Model file for the job. Use its own axes, mm. Face numbers are marked on the shaded views. Give positions to 0.01 mm unless a question says otherwise; leave off trailing zeros. Write each loop counter-clockwise with the first axis right and the second up, starting at its lowest first coordinate (ties: lowest second). Pieces come first, ordered by that corner, then holes. Notation, with made-up numbers: (-20, -15.75) - (15, -15.75) arc R27 ccw to (15, 10.25) - close; hole circle Ø9 at (0, 83). An arc over 180 degrees is marked (long way). Use CSV: the item, a comma, the result in double quotes.
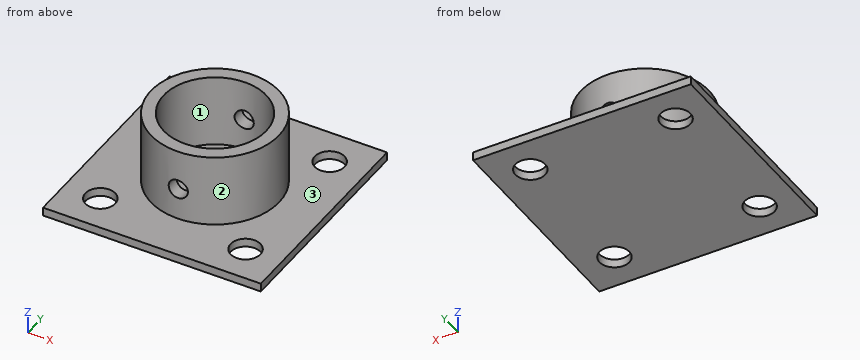
from build123d import *

# Parameters (mm, degrees)
F0_W     = 51
F0_H     = 51
F0_R     = 3.5
F1_DEPTH = 2
F2_R     = 15
F2_R_2   = 12
F3_DEPTH = 17
F4_W     = 51
F4_H     = 2.453923
F5_DEPTH = 17
F6_R     = 2.25
F7_DEPTH = 51.001
F8_W     = 51
F8_H     = 2.453923
F9_DEPTH = 17


with BuildPart() as f1:
    # F0 (on Top) → F1 (new body)
    with BuildSketch(Plane.XY):
        with Locations((-30.284861, 20.886204)):
            Rectangle(F0_W, F0_H)
        with Locations((-47.284861, 3.886204)):
            Circle(F0_R, mode=Mode.SUBTRACT)
        with Locations((-13.284861, 3.886204)):
            Circle(F0_R, mode=Mode.SUBTRACT)
        with Locations((-47.284861, 37.886204)):
            Circle(F0_R, mode=Mode.SUBTRACT)
        with Locations((-13.284861, 37.886204)):
            Circle(F0_R, mode=Mode.SUBTRACT)
    extrude(amount=F1_DEPTH)

    # F2 (on face) → F3 (join)
    with BuildSketch(Plane.XY.offset(2)):
        with Locations((-30.284861, 20.886204)):
            Circle(F2_R)
        with Locations((-30.284861, 20.886204)):
            Circle(F2_R_2, mode=Mode.SUBTRACT)
    extrude(amount=F3_DEPTH)

    # F4 (on face) → F5 (join)
    with BuildSketch(Plane.XY.offset(2)):
        with Locations((-30.284861, -3.386834)):
            Rectangle(F4_W, F4_H)
    extrude(amount=F5_DEPTH)

    # F6 (on face) → F7 (cut, through all)
    with BuildSketch(Plane.XZ.offset(4.613796)):
        with Locations((-30.284861, 9.5)):
            Circle(F6_R)
    extrude(amount=-F7_DEPTH, mode=Mode.SUBTRACT)

    # F8 (on face) → F9 (cut)
    with BuildSketch(Plane.XY.offset(19)):
        with Locations((-30.284861, -3.386834)):
            Rectangle(F8_W, F8_H)
    extrude(amount=-F9_DEPTH, mode=Mode.SUBTRACT)


solid = f1.part
(1) Saw through at B-B, the plane z = 9.5. List the corners of the cut face in (x, y), then the cut area to 3 significant figures.
Checked values:
outline,"(-32.53, 6.06) - (-32.53, 9.1) arc R12 cw to (-32.53, 32.67) - (-32.53, 35.72) arc R15 ccw to start; (-28.03, 6.06) arc R15 ccw to (-28.03, 35.72) - (-28.03, 32.67) arc R12 cw to (-28.03, 9.1) - close"
area,"227 mm^2"
(2) Saw through at C-C, the plane y = 1. List the corners of the cut face in (x, z) (3 decimals).
Checked values:
outline,"(-55.785, 0) - (-49.265, 0) - (-49.265, 2) - (-55.785, 2) - close; (-45.305, 0) - (-15.265, 0) - (-15.265, 2) - (-45.305, 2) - close; (-11.305, 0) - (-4.785, 0) - (-4.785, 2) - (-11.305, 2) - close"
(3) Saw through at A-A, the plane x = -29. List the corners of the cut face in (y, z).
Checked values:
outline,"(-4.61, 0) - (46.39, 0) - (46.39, 2) - (35.83, 2) - (35.83, 7.65) - (32.82, 7.65) - (32.82, 2) - (8.96, 2) - (8.96, 7.65) - (5.94, 7.65) - (5.94, 2) - (-4.61, 2) - close; (5.94, 11.35) - (8.96, 11.35) - (8.96, 19) - (5.94, 19) - close; (32.82, 11.35) - (35.83, 11.35) - (35.83, 19) - (32.82, 19) - close"
(4) Flat gauge pins, fed straight in: P1, Ø8, axis at x = -32, z = 8.5, coming from the +Y side; P2, Ø11, axis at x = -47.28, y = 37.89, coming from the +Z side. Where does each tip first touch, or does it go through?
Checked values:
P1,"stops at y = 35.89"
P2,"stops at z = 2"
(5) Wall check: probe 1 along X at (y, z) = (28, 7.5); probe 2 along Y at (x, z) = (-25, 8.5); probe 3 along Y at (x, z) = (-39, 6.25). Give the ranges that are in metal, low to high. Write a range as [from, to].
Checked values:
probe 1,"x = [-43.49, -39.95], [-20.62, -17.08]"
probe 2,"y = [6.85, 10.11], [31.66, 34.92]"
probe 3,"y = [8.68, 12.64], [29.14, 33.09]"
(6) Saw through at D-D, the plane y = 30.5. List the corners of the cut face in (x, z).
Checked values:
outline,"(-55.78, 0) - (-4.78, 0) - (-4.78, 2) - (-18.77, 2) - (-18.77, 19) - (-23.1, 19) - (-23.1, 2) - (-37.47, 2) - (-37.47, 19) - (-41.8, 19) - (-41.8, 2) - (-55.78, 2) - close"
(7) Pull direction Y, two halves, no side cores. Call the marked faces 1, 2 and 3: released by +Y, released by -Y, zero draft, split by the parting line, or undercut.
Checked values:
face 1,"undercut"
face 2,"split by the parting line"
face 3,"zero draft"
